from build123d import *

# Parameters (mm, degrees)
SKETCH1_W           = 539.75
SKETCH1_H           = 508
BOSS_EXTRUDE1_DEPTH = 3.175
SKETCH2_R           = 2.54
SKETCH2_R_2         = 3.175
SKETCH2_W           = 234.95
SKETCH2_H           = 368.3
CUT_EXTRUDE1_DEPTH  = 44.45
SKETCH3_W           = 34.925
SKETCH3_H           = 127
CUT_EXTRUDE2_DEPTH  = 742.218013222
SKETCH4_R           = 1.8034
CUT_EXTRUDE3_DEPTH  = 742.218013222


with BuildPart() as part:
    # Sketch1 → Boss-Extrude1 (new body)
    with BuildSketch(Plane.XY):
        with Locations((269.875, 254)):
            Rectangle(SKETCH1_W, SKETCH1_H)
    extrude(amount=BOSS_EXTRUDE1_DEPTH)

    # Sketch2 → Cut-Extrude1 (cut)
    with BuildSketch(Plane(origin=(0, 0, 0), x_dir=(-1, 0, 0), z_dir=(0, 0, -1))):
        with Locations((-339.725, 45.085)):
            Circle(SKETCH2_R)
        with Locations((-85.725, 45.085)):
            Circle(SKETCH2_R)
        with Locations((-15.24, 365.76)):
            Circle(SKETCH2_R_2)
        with Locations((-339.725, 75.565)):
            Circle(SKETCH2_R)
        with Locations((-85.725, 75.565)):
            Circle(SKETCH2_R)
        with Locations((-212.725, 184.15)):
            Rectangle(SKETCH2_W, SKETCH2_H)
    extrude(amount=-CUT_EXTRUDE1_DEPTH, mode=Mode.SUBTRACT)

    # Sketch3 → Cut-Extrude2 (cut, through all)
    with BuildSketch(Plane(origin=(0, 0, 0), x_dir=(-1, 0, 0), z_dir=(0, 0, -1))):
        with Locations((-17.4625, 444.5)):
            Rectangle(SKETCH3_W, SKETCH3_H)
    extrude(amount=-CUT_EXTRUDE2_DEPTH, mode=Mode.SUBTRACT)

    # Sketch4 → Cut-Extrude3 (cut, through all)
    with BuildSketch(Plane(origin=(0, 0, 0), x_dir=(-1, 0, 0), z_dir=(0, 0, -1))):
        with Locations((-311.1754, 373.8372)):
            Circle(SKETCH4_R)
        with Locations((-295.3004, 373.8372)):
            Circle(SKETCH4_R)
        with Locations((-130.2004, 373.8372)):
            Circle(SKETCH4_R)
        with Locations((-114.3254, 373.8372)):
            Circle(SKETCH4_R)
    extrude(amount=-CUT_EXTRUDE3_DEPTH, mode=Mode.SUBTRACT)


solid = part.part
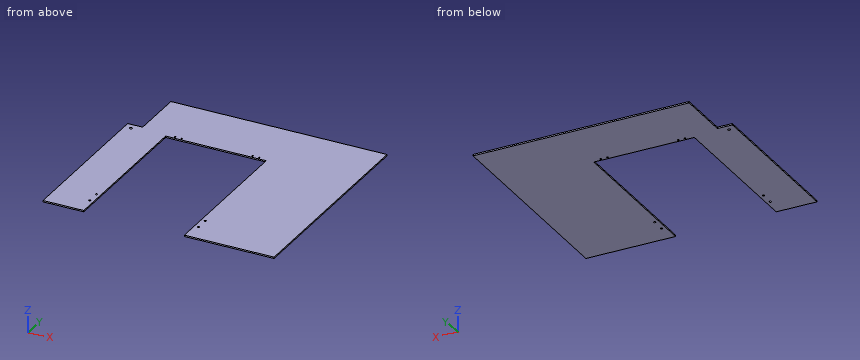
Geometry: final body of the model. Coordinates: model frame, mm. Give positions to 0.01 mm unless a question says otherwise; leave off trailing zeros. Loops run counter-clockwise (first coordinate to the right, second up) from the corner with the lowest first, then second, coordinate; pieces in that order, holes last. Notation, with made-up numbers: (-5, 50) - (4, 50) arc R18 cw to (4, 82) - close; hole circle Ø5 at (21, -7). An arc over 180 degrees is marked (long way). Answer as CSV lines item,"result". Start each with the question number.
1. Section D-D, the plane y = 470.5. Return loops of the section in (x, z) (3 decimals).
2. Section C-C, the plane x = 174. Return loops of the section in (y, z) (3 decimals), plus the area to 3 significant figures.
3. Section A-A, the plane y = 120. Return loops of the section in (x, z) (3 decimals).
4. Ray query, L1, parallel to X at y = 296, z = 0.7; L2, parallel to Y at x = 15.24, z = 2.55 (3 decimals); L3, parallel to Y at x = 280.5, z = 2.45. Return the intervals inside material, ascending.
5. Pin query (flat end, axial travel): P1, Ø12, axis at x = 307, y = 413.5, coming from the -Z side. Return the tip coordinate at first contact, or that it passes through.
6. Section B-B, the plane z = 2. Give the number of separate pieces and of enclosed holes in the cut face, plus the area to 3 significant figures.
Answers:
1,outline,"(34.925, 0) - (539.75, 0) - (539.75, 3.175) - (34.925, 3.175) - close"
2,outline,"(368.3, 0) - (508, 0) - (508, 3.175) - (368.3, 3.175) - close"
2,area,"444 mm2"
3,outline,"(0, 0) - (95.25, 0) - (95.25, 3.175) - (0, 3.175) - close; (330.2, 0) - (539.75, 0) - (539.75, 3.175) - (330.2, 3.175) - close"
4,L1,"x = 0 to 95.25, 330.2 to 539.75"
4,L2,"y = 0 to 362.585, 368.935 to 381"
4,L3,"y = 368.3 to 508"
5,P1,"stops at z = 0"
6,separate pieces,"1"
6,enclosed holes,"9"
6,area,"183,000 mm2"
